Model file for the job. Use its own axes, mm. Round coordinates to 2 decimals unless told otherwise and drop trailing zeros. Loops run counter-clockwise (first coordinate to the right, second up) from the corner with the lowest first, then second, coordinate; pieces in that order, holes last. Notation, with made-up numbers: M -21.75,65 L 12.25,65 A21 ccw 12.25,103 Z; hole C -27.5,20 d2. An arc over 180 degrees is marked long. Use a Markdown table: item, result. Add a question column.
Q1. Mould opens along X. For faces 1 (the face through (-1, 4, -46.99)), 2 (the face through (-81.1, 4.4, 35.2)), 3 (the face through (-37.333, 4.383, -42.694)), 4 (the face through (-110.48, 4.38, 1.03)) say: +X half, -X half, draft (parallel to the pull), parting line (faces both ways), or undercut.
Q2. Cut at A-A (z = 0). Give the cut face in (x, y), plus the area to 3 significant figures.
Q3. Cut at B-B (x = -12.7). Give the cut face in (y, z), plus the area to 3 significant figures.
Q4. Cut at D-D (z = -30). Give the cut face in (x, y).
Q5. Cut at C-C (y = 2). State how many separate pieces and enclosed holes the cut face has, plus the area to 3 significant figures.
Q6. Pin check, flat tips, straight feed: pin 1 (4 mm diameter, centred on y = 7.5, z = 29, fed in from +X); pin 2 (4 mm diameter, centred on x = -80, y = 7.5, fed in from +Z). Stop position of each tip, or through.
Q7. Probe line 1 (Z direction, x = -100, y = 2); line 2 (Z direction, x = 15, y = 7); line 3 (X direction, y = 8, z = -20.5). List the from-to ranges inside material, lowest first. Write a range as from..to.
from build123d import *

# Parameters (mm, degrees)
BOSS_EXTRUDE1_DEPTH = 8.89
SKETCH4_R           = 2.5527
CUT_EXTRUDE1_DEPTH  = 121.395732067


with BuildPart() as part:
    # Sketch1 → Boss-Extrude1 (new body)
    with BuildSketch(Plane(origin=(0, 0, 0), x_dir=(1, 0, 0), z_dir=(0, 1, 0))):
        with BuildLine():
            Line((-63.5, 46.99), (63.5, 46.99))
            ThreePointArc((63.5, 46.99), (110.49, 0), (63.5, -46.99))
            Line((63.5, -46.99), (-63.5, -46.99))
            ThreePointArc((-63.5, -46.99), (-110.49, 0), (-63.5, 46.99))
        make_face()
    extrude(amount=BOSS_EXTRUDE1_DEPTH)

    # Sketch4 → Cut-Extrude1 (cut, through all)
    with BuildSketch(Plane.XZ):
        with Locations(Location((83.6295, -34.865316731, 0), (0, 0, 270))):
            Circle(SKETCH4_R)
        with Locations(Location((63.5, -40.259, 0), (0, 0, 270))):
            Circle(SKETCH4_R)
        with Locations(Location((38.1, -40.259, 0), (0, 0, 270))):
            Circle(SKETCH4_R)
        with Locations(Location((12.7, -40.259, 0), (0, 0, 270))):
            Circle(SKETCH4_R)
        with Locations(Location((-12.7, -40.259, 0), (0, 0, 270))):
            Circle(SKETCH4_R)
        with Locations(Location((-38.1, -40.259, 0), (0, 0, 270))):
            Circle(SKETCH4_R)
        with Locations(Location((-63.5, -40.259, 0), (0, 0, 270))):
            Circle(SKETCH4_R)
        with Locations(Location((-83.6295, -34.865316731, 0), (0, 0, 270))):
            Circle(SKETCH4_R)
        with Locations(Location((-98.365316731, -20.1295, 0), (0, 0, 270))):
            Circle(SKETCH4_R)
        with Locations(Location((-103.759, 0, 0), (0, 0, 270))):
            Circle(SKETCH4_R)
        with Locations(Location((-98.365316731, 20.1295, 0), (0, 0, 270))):
            Circle(SKETCH4_R)
        with Locations(Location((-83.6295, 34.865316731, 0), (0, 0, 270))):
            Circle(SKETCH4_R)
        with Locations(Location((-63.5, 40.259, 0), (0, 0, 270))):
            Circle(SKETCH4_R)
        with Locations(Location((-38.1, 40.259, 0), (0, 0, 270))):
            Circle(SKETCH4_R)
        with Locations(Location((-12.7, 40.259, 0), (0, 0, 270))):
            Circle(SKETCH4_R)
        with Locations(Location((12.7, 40.259, 0), (0, 0, 270))):
            Circle(SKETCH4_R)
        with Locations(Location((38.1, 40.259, 0), (0, 0, 270))):
            Circle(SKETCH4_R)
        with Locations(Location((63.5, 40.259, 0), (0, 0, 270))):
            Circle(SKETCH4_R)
        with Locations(Location((83.6295, 34.865316731, 0), (0, 0, 270))):
            Circle(SKETCH4_R)
        with Locations(Location((98.365316731, 20.1295, 0), (0, 0, 270))):
            Circle(SKETCH4_R)
        with Locations(Location((103.759, 0, 0), (0, 0, 270))):
            Circle(SKETCH4_R)
        with Locations(Location((98.365316731, -20.1295, 0), (0, 0, 270))):
            Circle(SKETCH4_R)
    extrude(amount=-CUT_EXTRUDE1_DEPTH, mode=Mode.SUBTRACT)


solid = part.part
Checked values:
| question | item | result |
|---|---|---|
| 1 | face 1 | draft |
| 1 | face 2 | undercut |
| 1 | face 3 | undercut |
| 1 | face 4 | -X half |
| 2 | outline | M -110.49,0 L -106.31,0 L -106.31,8.89 L -110.49,8.89 Z; M -101.21,0 L 101.21,0 L 101.21,8.89 L -101.21,8.89 Z; M 106.31,0 L 110.49,0 L 110.49,8.89 L 106.31,8.89 Z |
| 2 | area | 1,870 mm^2 |
| 3 | outline | M 0,-46.99 L 8.89,-46.99 L 8.89,-42.81 L 0,-42.81 Z; M 0,-37.71 L 8.89,-37.71 L 8.89,37.71 L 0,37.71 Z; M 0,42.81 L 8.89,42.81 L 8.89,46.99 L 0,46.99 Z |
| 3 | area | 745 mm^2 |
| 4 | outline | M -99.67,0 L 99.67,0 L 99.67,8.89 L -99.67,8.89 Z |
| 5 | separate pieces | 1 |
| 5 | enclosed holes | 22 |
| 5 | area | 18,400 mm^2 |
| 6 | pin 1 | stops at x = 101.96 |
| 6 | pin 2 | stops at z = 44.7 |
| 7 | line 1 | z = -29.59..-22.09, -18.17..18.17, 22.09..29.59 |
| 7 | line 2 | z = -46.99..-41.37, -39.15..39.15, 41.37..46.99 |
| 7 | line 3 | x = -105.78..-100.89, -95.84..95.84, 100.89..105.78 |
